The model under review builds one solid part; all positions refer to its coordinate system, in mm. A direction names the side the tool comes from. Coordinates: 2 decimals unless noted, no trailing zeros. Write each loop counter-clockwise with the first axis right and the second up, starting at its lowest first coordinate (ties: lowest second). Pieces come first, ordered by that corner, then holes.
1) For P1, Ø10, axis at x = -6, y = 19.5, coming from the +Z side; P2, Ø2.5, axis at x = 9, z = -10.5, coming from the -Y side; P3, Ø1.9, axis at y = 2, z = 0, coming from the -X side (3 decimals), all flat-tipped, find the tip position at first contact; note any pin that passes through.
2) Mouldability with a two-part tool opening along X and no side actions: class faces 5 (the cylindrical face through (5.407, 79.66, 17.169)), 6 (the flat face through (-2.75, 2, -16)), 7 (the flat face through (-15.3, 36.6, -9.8)) as released by +X, released by -X, zero draft, split by the parting line, or undercut.
3) For line 1 (Y direction, x = -8, z = -14); line 2 (Y direction, x = 9.5, z = 11); line 3 (X direction, y = 5, z = -9.5), list the stretches that pass through material, from the lowest coordinate up.
4) Add section A-A, the plane y = 82.5. State the section outline as (x, z) points.
5) Machinability: for faces 1 (the flat face through (15.3, 89.8, -9.8)), 2 (the flat face through (0, 0.5, 13)), 3 (the flat face through (-15, 3.5, 0)), 4 (the flat face through (0, -1.3, 5)), which of the approach directions +Z, -Z, +X, -X, +Y, -Y give a long, thin tool a straight path to every point of the face, cutting with its end or side? Answer none if there is none.
from build123d import *

# Parameters (mm, degrees)
SKETCH1_R           = 18
BOSS_EXTRUDE1_DEPTH = 89.8
SKETCH2_R           = 18.65
BOSS_EXTRUDE2_DEPTH = 18
BOSS_EXTRUDE4_DEPTH = 1.3
BOSS_EXTRUDE3_START = 33.2
SKETCH3_R           = 18.65
BOSS_EXTRUDE3_DEPTH = 33.2
SKETCH11_R          = 4
CUT_EXTRUDE1_DEPTH  = 10.3
CUT_EXTRUDE2_START  = -6.7
CUT_EXTRUDE2_DEPTH  = 6.7
SKETCH14_R          = 1.5
CUT_EXTRUDE3_DEPTH  = 10
SKETCH16_R          = 18.025
BOSS_EXTRUDE5_DEPTH = 20.5
SKETCH17_R          = 19.645678417
SKETCH17_R_2        = 17.75
CUT_EXTRUDE5_DEPTH  = 0.5
CUT_EXTRUDE6_DEPTH  = 3.5
SKETCH19_R          = 2.375
BOSS_EXTRUDE6_DEPTH = 3
CUT_EXTRUDE7_DEPTH  = 3


with BuildPart() as part:
    # Sketch1 → Boss-Extrude1 (new body)
    with BuildSketch(Plane(origin=(0, 0, 0), x_dir=(1, 0, 0), z_dir=(0, 1, 0))):
        with Locations(Location((0, 0, 0), (0, 0, 270))):
            Circle(SKETCH1_R)
    extrude(amount=BOSS_EXTRUDE1_DEPTH)

    # Sketch2 → Boss-Extrude2 (add)
    with BuildSketch(Plane(origin=(0, 89.8, 0), x_dir=(1, 0, 0), z_dir=(0, 1, 0))):
        with Locations(Location((0, 0, 0), (0, 0, 270))):
            Circle(SKETCH2_R)
    extrude(amount=BOSS_EXTRUDE2_DEPTH)

    # Sketch9 → Boss-Extrude4 (add)
    with BuildSketch(Plane.XZ):
        with BuildLine():
            Line((4.582575695, -10), (-4.582575695, -10))
            ThreePointArc((-4.582575695, -10), (-11, 0), (-4.582575695, 10))
            Line((-4.582575695, 10), (4.582575695, 10))
            ThreePointArc((4.582575695, 10), (11, 0), (4.582575695, -10))
        make_face()
    extrude(amount=BOSS_EXTRUDE4_DEPTH)

    # Sketch3 → Boss-Extrude3 (add)
    with BuildSketch(Plane(origin=(0, 69.8, 0), x_dir=(-1, 0, 0), z_dir=(0, -1, 0)).offset(BOSS_EXTRUDE3_START)):
        with Locations(Location((0, 0, 0), (0, 0, 270))):
            Circle(SKETCH3_R)
    extrude(amount=-BOSS_EXTRUDE3_DEPTH)

    # Sketch11 → Cut-Extrude1 (cut)
    with BuildSketch(Plane.XZ.offset(1.3)):
        with Locations(Location((0, 0, 0), (0, 0, 270))):
            Circle(SKETCH11_R)
    extrude(amount=-CUT_EXTRUDE1_DEPTH, mode=Mode.SUBTRACT)

    # Sketch13 → Cut-Extrude2 (cut)
    with BuildSketch(Plane(origin=(0, 107.8, 0), x_dir=(1, 0, 0), z_dir=(0, 1, 0)).offset(CUT_EXTRUDE2_START)):
        with BuildLine():
            Line((-16.522711642, -8.65), (16.522711642, -8.65))
            ThreePointArc((16.522711642, -8.65), (0, -18.65), (-16.522711642, -8.65))
        make_face()
    extrude(amount=CUT_EXTRUDE2_DEPTH, mode=Mode.SUBTRACT)

    # Sketch14 → Cut-Extrude3 (cut)
    with BuildSketch(Plane.XZ):
        with Locations(Location((-9.899494937, 9.899494937, 0), (0, 0, 270))):
            Circle(SKETCH14_R)
        with Locations(Location((9.899494937, 9.899494937, 0), (0, 0, 270))):
            Circle(SKETCH14_R)
        with Locations(Location((9.899494937, -9.899494937, 0), (0, 0, 270))):
            Circle(SKETCH14_R)
        with Locations(Location((-9.899494937, -9.899494937, 0), (0, 0, 270))):
            Circle(SKETCH14_R)
    extrude(amount=-CUT_EXTRUDE3_DEPTH, mode=Mode.SUBTRACT)

    # Sketch16 → Boss-Extrude5 (add)
    with BuildSketch(Plane(origin=(0, 6.5, 0), x_dir=(-1, 0, 0), z_dir=(0, -1, 0))):
        with Locations(Location((0, 0, 0), (0, 0, 90))):
            Circle(SKETCH16_R)
    extrude(amount=-BOSS_EXTRUDE5_DEPTH)

    # Sketch17 → Cut-Extrude5 (cut)
    with BuildSketch(Plane(origin=(0, 31.5, 0), x_dir=(-1, 0, 0), z_dir=(0, -1, 0))):
        Circle(SKETCH17_R)
        with Locations(Location((0, 0, 0), (0, 0, 90))):
            Circle(SKETCH17_R_2, mode=Mode.SUBTRACT)
    extrude(amount=-CUT_EXTRUDE5_DEPTH, mode=Mode.SUBTRACT)

    # Sketch18 → Cut-Extrude6 (cut)
    with BuildSketch(Plane.XZ):
        with BuildLine():
            Line((2.75, -15), (2.75, -20))
            Line((2.75, -20), (-2.75, -20))
            Line((-2.75, -20), (-2.75, -15))
            ThreePointArc((-2.75, -15), (0, -12.25), (2.75, -15))
        make_face()
        with BuildLine():
            Line((2.75, 15), (2.75, 20))
            Line((2.75, 20), (-2.75, 20))
            Line((-2.75, 20), (-2.75, 15))
            ThreePointArc((-2.75, 15), (0, 12.25), (2.75, 15))
        make_face()
        with BuildLine():
            Line((-15, 2.75), (-20, 2.75))
            Line((-20, 2.75), (-20, -2.75))
            Line((-20, -2.75), (-15, -2.75))
            ThreePointArc((-15, -2.75), (-12.25, 0), (-15, 2.75))
        make_face()
        with BuildLine():
            Line((15, -2.75), (20, -2.75))
            Line((20, -2.75), (20, 2.75))
            Line((20, 2.75), (15, 2.75))
            ThreePointArc((15, 2.75), (12.25, 0), (15, -2.75))
        make_face()
    extrude(amount=-CUT_EXTRUDE6_DEPTH, mode=Mode.SUBTRACT)

    # Sketch19 → Boss-Extrude6 (add)
    with BuildSketch(Plane.XZ.offset(-3.5)):
        with Locations(Location((-15, 0, 0), (0, 0, 270))):
            Circle(SKETCH19_R)
        with Locations(Location((0, 15, 0), (0, 0, 270))):
            Circle(SKETCH19_R)
        with Locations(Location((15, 0, 0), (0, 0, 270))):
            Circle(SKETCH19_R)
        with Locations(Location((0, -15, 0), (0, 0, 270))):
            Circle(SKETCH19_R)
    extrude(amount=BOSS_EXTRUDE6_DEPTH)

    # Sketch20 → Cut-Extrude7 (cut)
    with BuildSketch(Plane.XZ.offset(-0.5)):
        Polygon((16.515813069, 0.875155083), (15, 1.750310167), (13.484186931, 0.875155083), (13.484186931, -0.875155083), (15, -1.750310167), (16.515813069, -0.875155083), align=None)
        Polygon((-1.750310167, 15), (-0.875155083, 13.484186931), (0.875155083, 13.484186931), (1.750310167, 15), (0.875155083, 16.515813069), (-0.875155083, 16.515813069), align=None)
        Polygon((0.875155083, -16.515813069), (1.750310167, -15), (0.875155083, -13.484186931), (-0.875155083, -13.484186931), (-1.750310167, -15), (-0.875155083, -16.515813069), align=None)
        Polygon((-16.515813069, -0.875155083), (-15, -1.750310167), (-13.484186931, -0.875155083), (-13.484186931, 0.875155083), (-15, 1.750310167), (-16.515813069, 0.875155083), align=None)
    extrude(amount=-CUT_EXTRUDE7_DEPTH, mode=Mode.SUBTRACT)


solid = part.part
Geometry results:
1. P1: stops at z = 18
1. P2: stops at y = 0
1. P3: stops at x = -17.375
2. face 5: split by the parting line
2. face 6: undercut
2. face 7: zero draft
3. line 1: y = 0 to 107.8
3. line 2: y = 6.5 to 101.1
3. line 3: x = -15.29 to -11.35, -8.45 to 8.45, 11.35 to 15.29
4. outline: circle Ø36 at (0, 0)
5. face 1: none
5. face 2: +Z, -Y
5. face 3: -Y
5. face 4: +Z, -Z, +X, -X, -Y
